Check sheet for the modelled part. Datum: model origin and axes. Units: mm. Face numbers are marked on the shaded views. A direction names the side the tool comes from. Give positions to 0.01 mm unless a question says otherwise; leave off trailing zeros. Order: outer loops, then holes, each group sorted by start corner. A loop starts at its lowest first (then second) coordinate and runs counter-clockwise, first axis right, second up. Notation, with made-up numbers: (32, -3.75) -> (37, -3.75) arc R25 ccw to (37, 31.25) -> close; hole circle Ø2 at (-8, -29). An arc over 180 degrees is marked (long way). Write each question's results on one line, items separated by ' | '.
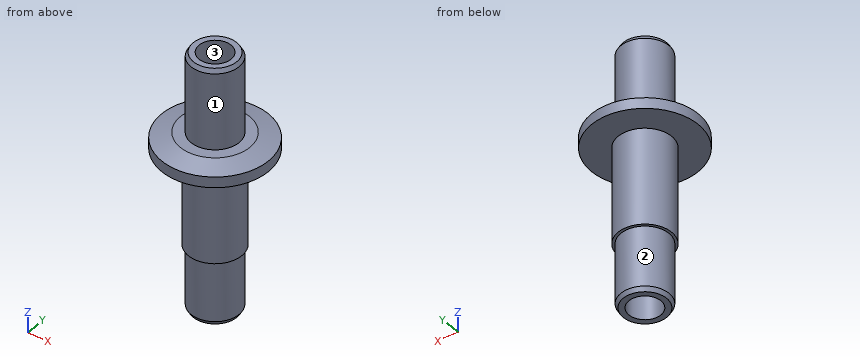
from build123d import *

# Parameters (mm, degrees)
F0_R      = 4.5
F1_DEPTH  = 12
F2_R      = 5
F3_DEPTH  = 18
F4_R      = 10
F5_DEPTH  = 3
F6_R      = 4.5
F7_DEPTH  = 15
F8_R      = 3
F9_DEPTH  = 48.001
F10_SIZE2 = 0.4330127019
F10_SIZE  = 0.75
F11_SIZE2 = 0.4330127019
F11_SIZE  = 0.75
F12_SIZE2 = 3.4874144438
F12_SIZE  = 1


with BuildPart() as f1:
    # F0 (on Top) → F1 (new body)
    with BuildSketch(Plane.XY):
        Circle(F0_R)
    extrude(amount=F1_DEPTH)

    # F2 (on face) → F3 (join)
    with BuildSketch(Plane.XY.offset(12)):
        Circle(F2_R)
    extrude(amount=F3_DEPTH)

    # F4 (on face) → F5 (join)
    with BuildSketch(Plane.XY.offset(30)):
        Circle(F4_R)
    extrude(amount=F5_DEPTH)

    # F6 (on face) → F7 (join)
    with BuildSketch(Plane.XY.offset(33)):
        Circle(F6_R)
    extrude(amount=F7_DEPTH)

    # F8 (on face) → F9 (cut, through all)
    with BuildSketch(Plane(origin=(0, 0, 0), x_dir=(1, 0, 0), z_dir=(0, 0, -1))):
        Circle(F8_R)
    extrude(amount=-F9_DEPTH, mode=Mode.SUBTRACT)

    # F10
    f10_edges = [f1.edges().sort_by_distance(p)[0] for p in [
        (-4.5, 0, 48),
    ]]
    f10_side = f1.faces().sort_by_distance((-4.5, 0, 40.5))[0]
    chamfer(f10_edges, length=F10_SIZE, length2=F10_SIZE2, reference=f10_side)

    # F11
    f11_edges = [f1.edges().sort_by_distance(p)[0] for p in [
        (-4.5, 0, 0),
    ]]
    f11_side = f1.faces().sort_by_distance((-4.5, 0, 6))[0]
    chamfer(f11_edges, length=F11_SIZE, length2=F11_SIZE2, reference=f11_side)

    # F12
    f12_edges = [f1.edges().sort_by_distance(p)[0] for p in [
        (-10, 0, 33),
    ]]
    f12_side = f1.faces().sort_by_distance((-10, 0, 31.5))[0]
    chamfer(f12_edges, length=F12_SIZE, length2=F12_SIZE2, reference=f12_side)


solid = f1.part
1. Section check A-A on y = 0. Record the cut outline in (x, z).
Verdict:
outline: (-10, 30) -> (-5, 30) -> (-5, 12) -> (-4.5, 12) -> (-4.5, 0.75) -> (-4.07, 0) -> (-3, 0) -> (-3, 48) -> (-4.07, 48) -> (-4.5, 47.25) -> (-4.5, 33) -> (-6.51, 33) -> (-10, 32) -> close; (3, 0) -> (4.07, 0) -> (4.5, 0.75) -> (4.5, 12) -> (5, 12) -> (5, 30) -> (10, 30) -> (10, 32) -> (6.51, 33) -> (4.5, 33) -> (4.5, 47.25) -> (4.07, 48) -> (3, 48) -> close
2. Material ranges on probe 1 along Y at (x, z) = (0, 22); probe 2 along Z at (x, y) = (-6.25, -0.25); probe 3 along Y at (x, z) = (-0.5, 34), recorded low to high. Write a range as from..to.
Verdict:
probe 1: y = -5..-3, 3..5 | probe 2: z = 30..33 | probe 3: y = -4.47..-2.96, 2.96..4.47
3. Access from +Z, -Z, +X, -X, +Y, -Y to the whole of each face (thin tool, end or side, straight path). Record for the marked faces 1, 2 and 3.
Verdict:
face 1: +Z | face 2: -Z | face 3: +Z, -Z
4. Gauge pin test, flat ends, axial feed: pin 1 Ø4 at (y, z) = (4.5, 9) entering from -X; pin 2 Ø8 at (y, z) = (-4, 7.5) entering from +X; pin 3 Ø8 at (x, z) = (7, 26.5) entering from -Y. Record the tip position at first contact, or that the pin passes through.
Verdict:
pin 1: stops at x = -3.74 | pin 2: stops at x = 4.5 | pin 3: stops at y = -8.62
5. Section check C-C on z = 44. Record the cut outline in (x, y), then the cut area to 3 significant figures.
Verdict:
outline: circle Ø9 at (0, 0); hole circle Ø6 at (0, 0) | area: 35.3 mm^2
6. Section check B-B on z = 23. Record the cut outline in (x, y), then the cut area to 3 significant figures.
Verdict:
outline: circle Ø10 at (0, 0); hole circle Ø6 at (0, 0) | area: 50.3 mm^2
